from build123d import *

# Parameters (mm, degrees)
SKETCH1_R           = 1
SKETCH1_R_2         = 4
BOSS_EXTRUDE1_DEPTH = 3
SKETCH2_W           = 2.5
SKETCH2_H           = 22
BOSS_EXTRUDE2_DEPTH = 14
SKETCH4_R           = 4.6
CUT_EXTRUDE2_DEPTH  = 1.2
SKETCH5_R           = 1.9
CUT_EXTRUDE3_DEPTH  = 1.5


with BuildPart() as part:
    # Sketch1 → Boss-Extrude1 (new body)
    with BuildSketch(Plane(origin=(0, 0, 0), x_dir=(1, 0, 0), z_dir=(0, 1, 0))):
        with BuildLine():
            Line((-14, -11), (-14, 11))
            Line((-14, 11), (6, 11))
            ThreePointArc((6, 11), (17, 0), (6, -11))
            Line((6, -11), (-14, -11))
        make_face()
        with Locations((6, -7)):
            Circle(SKETCH1_R, mode=Mode.SUBTRACT)
        with Locations((-1, 0)):
            Circle(SKETCH1_R, mode=Mode.SUBTRACT)
        with Locations((6, 0)):
            Circle(SKETCH1_R_2, mode=Mode.SUBTRACT)
        with Locations((13, 0)):
            Circle(SKETCH1_R, mode=Mode.SUBTRACT)
        with Locations((6, 7)):
            Circle(SKETCH1_R, mode=Mode.SUBTRACT)
    extrude(amount=BOSS_EXTRUDE1_DEPTH)

    # Sketch2 → Boss-Extrude2 (add)
    with BuildSketch(Plane(origin=(0, 3, 0), x_dir=(1, 0, 0), z_dir=(0, 1, 0))):
        with Locations((-12.75, 0)):
            Rectangle(SKETCH2_W, SKETCH2_H)
    extrude(amount=BOSS_EXTRUDE2_DEPTH)

    # Sketch4 → Cut-Extrude2 (cut)
    with BuildSketch(Plane.XZ):
        with Locations((6, 0)):
            Circle(SKETCH4_R)
    extrude(amount=-CUT_EXTRUDE2_DEPTH, mode=Mode.SUBTRACT)

    # Sketch5 → Cut-Extrude3 (cut)
    with BuildSketch(Plane.XZ):
        with Locations((13, 0)):
            Circle(SKETCH5_R)
        with Locations((6, -7)):
            Circle(SKETCH5_R)
        with Locations((-1, 0)):
            Circle(SKETCH5_R)
        with Locations((6, 7)):
            Circle(SKETCH5_R)
    extrude(amount=-CUT_EXTRUDE3_DEPTH, mode=Mode.SUBTRACT)


solid = part.part
For this review, take the finished solid that the model builds, in its own axes (mm). A direction names the side the tool comes from. Coordinates: 2 decimals unless noted, no trailing zeros. Loops run counter-clockwise (first coordinate to the right, second up) from the corner with the lowest first, then second, coordinate; pieces in that order, holes last. Notation, with made-up numbers: (77, 72.25) - (117, 72.25) arc R23 cw to (117, 91.25) - close; hole circle Ø6 at (43, 53). An arc over 180 degrees is marked (long way). Use a Markdown table: item, result. Add a question column.
Item 1: We need section B-B (y = 2.5). Give the boundary of the cut face in (x, z).
Item 2: We need section C-C (z = 0). Give the number of separate pieces and of enclosed holes in the cut face, and give its area (3 significant figures).
Item 3: We need section A-A (x = -1). Give the boundary of the cut face in (y, z).
Item 4: For line 1 (Z direction, x = 6, y = 0.65); line 2 (Z direction, x = -1, y = 2); line 3 (X direction, y = 2.15, z = 0), list the stretches that pass through material, from the lowest coordinate up.
Item 5: Mouldability with a two-part tool opening along Z and no side actions: class faces 4 (the face through (-2, 0, -3)), 5 (the face through (4.6, 0.74, 8.284)), 6 (the face through (-6.3, 2.8, -11)) as pulls with the +Z half, pulls with the -Z half, needs draft (parallel to the pull), parting line crosses it, or undercut.
Item 6: We need section D-D (z = 7). Give the boundary of the cut face in (x, y).
Item 7: Insertion check: pin 1 Ø5 at (y, z) = (9, -3) entering from +X; pin 2 Ø4 at (x, z) = (5.5, 7) entering from -Y; pin 3 Ø3 at (x, z) = (13, 0) entering from +Y; pin 4 Ø1.1 at (x, z) = (5.5, -8) entering from -Y. Each pin has a flat end and moves straight along its axis. Give the tip position at first contact, or say it passes through.
Item 8: Tool access review of faces 1 (the face through (0.812, 0.74, 0.571)), 2 (the face through (3, 3, -3)), 3 (the face through (-13, 17, 0)): name each direction out of +Z, -Z, +X, -X, +Y, -Y from which nothing blocks a thin tool from reaching the whole face with its end or side.
Results list:
| question | item | result |
|---|---|---|
| 1 | outline | (-14, -11) - (6, -11) arc R11 ccw to (6, 11) - (-14, 11) - close; hole circle Ø2 at (-1, 0); hole circle Ø8 at (6, 0); hole circle Ø2 at (6, -7); hole circle Ø2 at (6, 7); hole circle Ø2 at (13, 0) |
| 2 | separate pieces | 4 |
| 2 | enclosed holes | 0 |
| 2 | area | 85.2 mm^2 |
| 3 | outline | (0, -11) - (3, -11) - (3, -1) - (1.5, -1) - (1.5, -1.9) - (0, -1.9) - close; (0, 1.9) - (1.5, 1.9) - (1.5, 1) - (3, 1) - (3, 11) - (0, 11) - close |
| 4 | line 1 | z = -11 to -8.9, -5.1 to -4.6, 4.6 to 5.1, 8.9 to 11 |
| 4 | line 2 | z = -11 to -1, 1 to 11 |
| 4 | line 3 | x = -14 to -2, 0 to 2, 10 to 12, 14 to 17 |
| 5 | face 4 | needs draft |
| 5 | face 5 | undercut |
| 5 | face 6 | pulls with the -Z half |
| 6 | outline | (-14, 0) - (4.1, 0) - (4.1, 1.5) - (5, 1.5) - (5, 3) - (-11.5, 3) - (-11.5, 17) - (-14, 17) - close; (7, 1.5) - (7.9, 1.5) - (7.9, 0) - (14.49, 0) - (14.49, 3) - (7, 3) - close |
| 7 | pin 1 | stops at x = -11.5 |
| 7 | pin 2 | stops at y = 0 |
| 7 | pin 3 | stops at y = 3 |
| 7 | pin 4 | stops at y = 1.5 |
| 8 | face 1 | -Y |
| 8 | face 2 | +Z, -Z, +X, +Y |
| 8 | face 3 | +Z, -Z, +X, -X, +Y |
